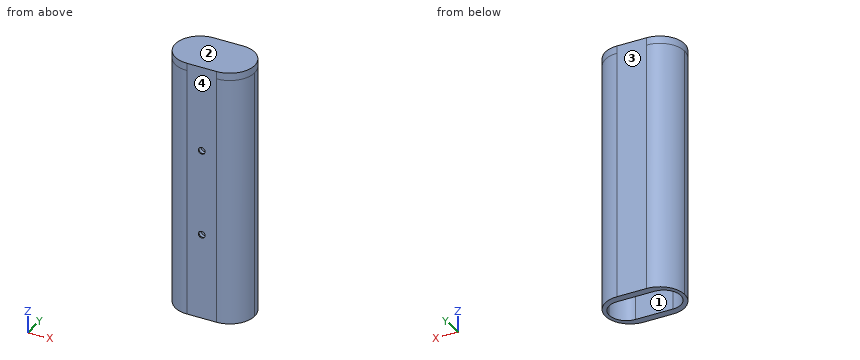
```python
from build123d import *

# Parameters (mm, degrees)
BOSS_EXTRUDE1_DEPTH = 168.91
BOSS_EXTRUDE2_DEPTH = 5.08
SKETCH5_R           = 3.683
CUT_EXTRUDE2_DEPTH  = 4.191
SKETCH6_R           = 2.286
CUT_EXTRUDE3_DEPTH  = 6.731


with BuildPart() as part:
    # Sketch1 → Boss-Extrude1 (new body)
    with BuildSketch(Plane.XY):
        with BuildLine():
            ThreePointArc((-24.13, 0), (-20.74503307, 8.17203307), (-12.573, 11.557))
            Line((-12.573, 11.557), (12.573, 11.557))
            ThreePointArc((12.573, 11.557), (20.74503307, 8.17203307), (24.13, 0))
            Line((24.13, 0), (26.67, 0))
            ThreePointArc((26.67, 0), (21.797135519, 11.764135519), (10.033, 16.637))
            Line((10.033, 16.637), (-10.033, 16.637))
            ThreePointArc((-10.033, 16.637), (-21.797135519, 11.764135519), (-26.67, 0))
            Line((-26.67, 0), (-24.13, 0))
        make_face()
        with BuildLine():
            ThreePointArc((-12.573, -11.557), (-20.74503307, -8.17203307), (-24.13, 0))
            Line((-24.13, 0), (-26.67, 0))
            ThreePointArc((-26.67, 0), (-21.797135519, -11.764135519), (-10.033, -16.637))
            Line((-10.033, -16.637), (10.033, -16.637))
            ThreePointArc((10.033, -16.637), (21.797135519, -11.764135519), (26.67, 0))
            Line((26.67, 0), (24.13, 0))
            ThreePointArc((24.13, 0), (20.74503307, -8.17203307), (12.573, -11.557))
            Line((12.573, -11.557), (-12.573, -11.557))
        make_face()
    extrude(amount=-BOSS_EXTRUDE1_DEPTH)

    # Sketch3 → Boss-Extrude2 (add)
    with BuildSketch(Plane.XY):
        with BuildLine():
            Line((-10.033, 16.637), (10.033, 16.637))
            ThreePointArc((10.033, 16.637), (26.67, 0), (10.033, -16.637))
            Line((10.033, -16.637), (-10.033, -16.637))
            ThreePointArc((-10.033, -16.637), (-26.67, 0), (-10.033, 16.637))
        make_face()
    extrude(amount=BOSS_EXTRUDE2_DEPTH)

    # Sketch5 → Cut-Extrude2 (cut)
    with BuildSketch(Plane(origin=(0, -11.557, 0), x_dir=(1, 0, 0), z_dir=(0, 1, 0))):
        with Locations((0, 110.998)):
            Circle(SKETCH5_R)
        with Locations((0, 52.832)):
            Circle(SKETCH5_R)
    extrude(amount=-CUT_EXTRUDE2_DEPTH, mode=Mode.SUBTRACT)

    # Sketch6 → Cut-Extrude3 (cut)
    with BuildSketch(Plane(origin=(0, -11.557, 0), x_dir=(1, 0, 0), z_dir=(0, 1, 0))):
        with Locations((0, 110.998)):
            Circle(SKETCH6_R)
        with Locations((0, 52.832)):
            Circle(SKETCH6_R)
    extrude(amount=-CUT_EXTRUDE3_DEPTH, mode=Mode.SUBTRACT)


solid = part.part
```
The listing builds one solid part. Answer for the finished solid, in the listing's coordinates (mm). Face numbers are marked on the shaded views. Round coordinates to 2 decimals unless told otherwise and drop trailing zeros. Write each loop counter-clockwise with the first axis right and the second up, starting at its lowest first coordinate (ties: lowest second). Pieces come first, ordered by that corner, then holes. Notation, with made-up numbers: (6.25, 40) -> (63.25, 40) arc R20 ccw to (63.25, 53) -> close; hole circle Ø10 at (-39.5, -31). An arc over 180 degrees is marked (long way). Write item = value, one per line.
1) Straight lines are drawn through the part: line 1 along Z through (x, y) = (0, -16.5); line 2 along Z through (x, y) = (0, -12.5) (3 decimals); line 3 along X through (y, z) = (0.5, -64). For each, find the intervals that lie inside material, in ascending order. Write a range as [from, to].
Check values:
line_1 = [-168.91, -113.28], [-108.71, -55.12], [-50.55, 5.08]
line_2 = [-168.91, -114.681], [-107.315, -56.515], [-49.149, 5.08]
line_3 = [-26.66, -24.12], [24.12, 26.66]
2) Section A-A on x = 0 is taken. Write down the section's boundary in (y, z) (3 decimals).
Check values:
outline = (-16.637, -168.91) -> (-11.557, -168.91) -> (-11.557, -114.681) -> (-15.748, -114.681) -> (-15.748, -113.284) -> (-16.637, -113.284) -> close; (-16.637, -108.712) -> (-15.748, -108.712) -> (-15.748, -107.315) -> (-11.557, -107.315) -> (-11.557, -56.515) -> (-15.748, -56.515) -> (-15.748, -55.118) -> (-16.637, -55.118) -> close; (-16.637, -50.546) -> (-15.748, -50.546) -> (-15.748, -49.149) -> (-11.557, -49.149) -> (-11.557, 0) -> (11.557, 0) -> (11.557, -168.91) -> (16.637, -168.91) -> (16.637, 5.08) -> (-16.637, 5.08) -> close
3) Section B-B on z = -88 is taken. Write down the section's boundary in (x, y).
Check values:
outline = (-10.03, -16.64) -> (10.03, -16.64) arc R16.64 ccw to (10.03, 16.64) -> (-10.03, 16.64) arc R16.64 ccw to start; hole (-12.57, -11.56) -> (12.57, -11.56) arc R11.56 ccw to (12.57, 11.56) -> (-12.57, 11.56) arc R11.56 ccw to start
4) For a pull along Y with two mould halves and no side action, classify the marked faces 1, 2, 3 and 4 as released by +Y, released by -Y, zero draft, split by the parting line, or undercut.
Check values:
face_1 = undercut
face_2 = zero draft
face_3 = released by +Y
face_4 = released by -Y
5) Section C-C on y = 7 is taken. Write down the section's boundary in (x, z).
Check values:
outline = (-25.13, -168.91) -> (-21.77, -168.91) -> (-21.77, 0) -> (21.77, 0) -> (21.77, -168.91) -> (25.13, -168.91) -> (25.13, 5.08) -> (-25.13, 5.08) -> close
6) Section D-D on x = -7 is taken. Write down the section's boundary in (y, z), plus the area to 3 significant figures.
Check values:
outline = (-16.64, -168.91) -> (-11.56, -168.91) -> (-11.56, 0) -> (11.56, 0) -> (11.56, -168.91) -> (16.64, -168.91) -> (16.64, 5.08) -> (-16.64, 5.08) -> close
area = 1,890 mm²
7) Given pin 1 (12 mm diameter, centred on x = -19, z = -39, fed in from -Y); pin 2 (10 mm diameter, centred on y = 10.5, z = -34.5, fed in from +X); pin 3 (3 mm diameter, centred on x = -7, y = -1.5, fed in from -Z); pin 4 (8 mm diameter, centred on y = -1.5, z = -125, fed in from +X), each flat-ended and moving along its own axis, determine where each tip first touches the part or whether it passes through.
Check values:
pin_1 = -16.37
pin_2 = 25.73
pin_3 = 0
pin_4 = 26.67
